Could you check a few things on this model? Use its own coordinates, in mm. A direction names the side the tool comes from. Give positions to 0.01 mm unless a question says otherwise; leave off trailing zeros. Order: outer loops, then holes, each group sorted by start corner. A loop starts at its lowest first (then second) coordinate and runs counter-clockwise, first axis right, second up. Notation, with made-up numbers: M -16,57.25 L 28,57.25 A29 ccw 28,96.25 Z; hole C 29,68.25 d8. An arc over 180 degrees is marked long. Use a Markdown table: item, result. Add a question column.
Item 1: Suppose I cut it at C-C on y = -6. Count the separate pieces of the cut face and the enclosed holes in it, plus the area to 3 significant figures.
Item 2: Suppose I cut it at B-B on z = 1.25. Write out the boundary of the cut face in (x, y).
Item 3: Suppose I cut it at A-A on x = -3. Write out the boundary of the cut face in (y, z).
Item 4: For faces 1 (the face through (-9.68, -11.43, 0.6)), 2 (the face through (47.18, -15.99, 0.57)), 3 (the face through (-23.5, -1.43, 2.49)), which set-ups out of +Z, -Z, +X, -X, +Y, -Y let a thin tool reach every point of the face, with its end or its side?
Item 5: If I drill on L1, parallel to Y at x = -3, z = 2.25; L2, parallel to Y at x = 51, z = 1.65; L3, parallel to Y at x = 28, z = 2.8, over which ranges is the centre line in solid material (lowest first)? Write a range as from..to.
Item 6: I'm going to push flat-ended pins straight in: pin 1 Ø1 at (x, z) = (44, 4) entering from +Y; pin 2 Ø4.5 at (x, y) = (-19, -6) entering from +Z; pin 3 Ø3 at (y, z) = (-3, 3) entering from -X. Where does each tip first touch, or does it pass through?
Item 7: If we mould it in two halves opening along X, with no side actions, what happens to faces 4 (the face through (-24.43, -5.99, 0.6)), 5 (the face through (56.685, -21.377, 0.57)), 6 (the face through (-12.6, -7.2, 2)), 7 (the face through (53.134, -22.157, 1.972))? For each: released by +X, released by -X, zero draft, split by the parting line, or undercut.
from build123d import *

# Parameters (mm, degrees)
F0_W         = 25
F0_H         = 12
F0_W_2       = 15
F1_DEPTH     = 5
F2_R         = 2
F3_DEPTH     = 5.001
F4_R         = 2
F5_T1_DEPTH  = 5
F5_T4_ANGLE  = 90
F5_T6_ANGLE  = 90
F5_T8_ANGLE  = 90
F5_T10_ANGLE = 90
F5_T12_ANGLE = 90
F5_T14_ANGLE = 90
F5_T16_ANGLE = 90
F5_T18_ANGLE = 90
F6_SIZE      = 1


# Not quite as in the source:
# - a fillet or chamfer that OpenCascade refuses, or shapes differently, is made with other operations: its cross-section is extruded or revolved along the edge and cut away or added


with BuildPart() as f1:
    # F0 (on Top) → F1 (new body)
    with BuildSketch(Plane.XY):
        with Locations((-12.5, -6)):
            Rectangle(F0_W, F0_H)
        Polygon((42.2861679354, -15.3909064497), (0, 0), (0, -12), (42.2861679354, -27.3909064497), align=None)
        with Locations((49.7861679354, -21.3909064497)):
            Rectangle(F0_W_2, F0_H)
    extrude(amount=F1_DEPTH)

    # F2 (on Top) → F3 (cut, through all)
    with BuildSketch(Plane.XY):
        with Locations((51.2861679354, -21.3909064497)):
            Circle(F2_R)
        with Locations((-19, -6)):
            Circle(F2_R)
        with Locations((43.2861679354, -21.3909064497)):
            Circle(F2_R)
        with Locations((-11, -6)):
            Circle(F2_R)
        with Locations((-3, -6)):
            Circle(F2_R)
    extrude(amount=F3_DEPTH, mode=Mode.SUBTRACT)

    # F4
    f4_edges = [f1.edges().sort_by_distance(p)[0] for p in [
        (21.143084, -19.695453, 5),
        (21.143084, -7.695453, 5),
        (-12.5, -12, 5),
        (-12.5, 0, 5),
        (49.786168, -27.390906, 5),
        (57.286168, -21.390906, 5),
        (49.786168, -15.390906, 5),
        (49.786168, -27.390906, 0),
        (21.143084, -19.695453, 0),
        (-12.5, -12, 0),
        (57.286168, -21.390906, 0),
        (21.143084, -7.695453, 0),
        (49.786168, -15.390906, 0),
        (-12.5, 0, 0),
        (-25, -6, 0),
        (-25, -6, 5),
    ]]
    fillet(f4_edges, radius=F4_R)

    # F5: fillet of radius 5 on 4 edges, made by hand

    # F5_s2 → F5_t1 (cut)
    with BuildSketch(Plane.XY):
        with BuildLine():
            ThreePointArc((52.2861679354, -15.3909064497), (55.8217018413, -16.8553725437), (57.2861679354, -20.3909064497))
            Line((57.2861679354, -20.3909064497), (57.2861679354, -15.3909064497))
            Line((57.2861679354, -15.3909064497), (52.2861679354, -15.3909064497))
        make_face()
        with BuildLine():
            ThreePointArc((-20, 0), (-23.5355339059, -1.4644660941), (-25, -5))
            Line((-25, -5), (-25, 0))
            Line((-25, 0), (-20, 0))
        make_face()
        with BuildLine():
            ThreePointArc((-25, -7), (-23.5355339059, -10.5355339059), (-20, -12))
            Line((-20, -12), (-25, -12))
            Line((-25, -12), (-25, -7))
        make_face()
        with BuildLine():
            ThreePointArc((57.2861679354, -22.3909064497), (55.8217018413, -25.9264403556), (52.2861679354, -27.3909064497))
            Line((52.2861679354, -27.3909064497), (57.2861679354, -27.3909064497))
            Line((57.2861679354, -27.3909064497), (57.2861679354, -22.3909064497))
        make_face()
    extrude(amount=F5_T1_DEPTH, mode=Mode.SUBTRACT)

    # F5_s3 → F5_t4 (revolve, cut)
    with BuildSketch(Plane.YZ.offset(52.2861679354)):
        with BuildLine():
            ThreePointArc((-25.3909064497, 5), (-26.805120012, 4.4142135624), (-27.3909064497, 3))
            Line((-27.3909064497, 3), (-27.3909064497, 5))
            Line((-27.3909064497, 5), (-25.3909064497, 5))
        make_face()
    revolve(axis=Axis((52.2861679354, -22.3909064497, 5), (0, 0, 1)), revolution_arc=F5_T4_ANGLE, mode=Mode.SUBTRACT)

    # F5_s5 → F5_t6 (revolve, cut)
    with BuildSketch(Plane.XZ.offset(7)):
        with BuildLine():
            ThreePointArc((-23, 5), (-24.4142135624, 4.4142135624), (-25, 3))
            Line((-25, 3), (-25, 5))
            Line((-25, 5), (-23, 5))
        make_face()
    revolve(axis=Axis((-20, -7, 5), (0, 0, 1)), revolution_arc=F5_T6_ANGLE, mode=Mode.SUBTRACT)

    # F5_s7 → F5_t8 (revolve, cut)
    with BuildSketch(Plane.YZ.offset(-20)):
        with BuildLine():
            ThreePointArc((-2, 5), (-0.5857864376, 4.4142135624), (0, 3))
            Line((0, 3), (0, 5))
            Line((0, 5), (-2, 5))
        make_face()
    revolve(axis=Axis((-20, -5, 5), (0, 0, 1)), revolution_arc=F5_T8_ANGLE, mode=Mode.SUBTRACT)

    # F5_s9 → F5_t10 (revolve, cut)
    with BuildSketch(Plane.XZ.offset(5)):
        with BuildLine():
            ThreePointArc((-23, 0), (-24.4142135624, 0.5857864376), (-25, 2))
            Line((-25, 2), (-25, 0))
            Line((-25, 0), (-23, 0))
        make_face()
    revolve(axis=Axis((-20, -5, 0), (0, 0, -1)), revolution_arc=F5_T10_ANGLE, mode=Mode.SUBTRACT)

    # F5_s11 → F5_t12 (revolve, cut)
    with BuildSketch(Plane.YZ.offset(-20)):
        with BuildLine():
            ThreePointArc((-10, 0), (-11.4142135624, 0.5857864376), (-12, 2))
            Line((-12, 2), (-12, 0))
            Line((-12, 0), (-10, 0))
        make_face()
    revolve(axis=Axis((-20, -7, 0), (0, 0, -1)), revolution_arc=F5_T12_ANGLE, mode=Mode.SUBTRACT)

    # F5_s13 → F5_t14 (revolve, cut)
    with BuildSketch(Plane.XZ.offset(22.3909064497)):
        with BuildLine():
            ThreePointArc((55.2861679354, 0), (56.7003814977, 0.5857864376), (57.2861679354, 2))
            Line((57.2861679354, 2), (57.2861679354, 0))
            Line((57.2861679354, 0), (55.2861679354, 0))
        make_face()
    revolve(axis=Axis((52.2861679354, -22.3909064497, 0), (0, 0, -1)), revolution_arc=F5_T14_ANGLE, mode=Mode.SUBTRACT)

    # F5_s15 → F5_t16 (revolve, cut)
    with BuildSketch(Plane.YZ.offset(52.2861679354)):
        with BuildLine():
            ThreePointArc((-17.3909064497, 0), (-15.9766928873, 0.5857864376), (-15.3909064497, 2))
            Line((-15.3909064497, 2), (-15.3909064497, 0))
            Line((-15.3909064497, 0), (-17.3909064497, 0))
        make_face()
    revolve(axis=Axis((52.2861679354, -20.3909064497, 0), (0, 0, -1)), revolution_arc=F5_T16_ANGLE, mode=Mode.SUBTRACT)

    # F5_s17 → F5_t18 (revolve, cut)
    with BuildSketch(Plane.XZ.offset(20.3909064497)):
        with BuildLine():
            ThreePointArc((55.2861679354, 5), (56.7003814977, 4.4142135624), (57.2861679354, 3))
            Line((57.2861679354, 3), (57.2861679354, 5))
            Line((57.2861679354, 5), (55.2861679354, 5))
        make_face()
    revolve(axis=Axis((52.2861679354, -20.3909064497, 5), (0, 0, 1)), revolution_arc=F5_T18_ANGLE, mode=Mode.SUBTRACT)

    # F6
    f6_edges = [f1.edges().sort_by_distance(p)[0] for p in [
        (-21, -6, 5),
        (-13, -6, 5),
        (-5, -6, 5),
        (41.286168, -21.390906, 5),
        (49.286168, -21.390906, 5),
    ]]
    chamfer(f6_edges, length=F6_SIZE)


solid = f1.part
Findings below:
| question | item | result |
|---|---|---|
| 1 | separate pieces | 4 |
| 1 | enclosed holes | 0 |
| 1 | area | 138 mm^2 |
| 2 | outline | M -24.85,-7 A4.85 ccw -20,-11.85 L 0.03,-11.85 L 42.31,-27.24 L 52.29,-27.24 A4.85 ccw 57.14,-22.39 L 57.14,-20.39 A4.85 ccw 52.29,-15.54 L 42.26,-15.54 L -0.03,-0.15 L -20,-0.15 A4.85 ccw -24.85,-5 Z; hole C -19,-6 d4; hole C -11,-6 d4; hole C -3,-6 d4; hole C 43.29,-21.39 d4; hole C 51.29,-21.39 d4 |
| 3 | outline | M -12,2 A2 ccw -10,0 L -8,0 L -8,4 L -9,5 L -10,5 A2 ccw -12,3 Z; M -4,0 L -2,0 A2 ccw 0,2 L 0,3 A2 ccw -2,5 L -3,5 L -4,4 Z |
| 4 | face 1 | -Z, -X, -Y |
| 4 | face 2 | -Z, +X, +Y |
| 4 | face 3 | +Z, -Z, -X, +Y |
| 5 | L1 | y = -12..-8, -4..0 |
| 5 | L2 | y = -27.36..-23.37, -19.41..-15.42 |
| 5 | L3 | y = -22.19..-10.19 |
| 6 | pin 1 | stops at y = -15.45 |
| 6 | pin 2 | stops at z = 4.25 |
| 6 | pin 3 | stops at x = -24.97 |
| 7 | face 4 | released by -X |
| 7 | face 5 | released by +X |
| 7 | face 6 | undercut |
| 7 | face 7 | undercut |
